Design review of the part built by this model. Coordinates are the model's own, in mm. A direction names the side the tool comes from. Give positions to 0.01 mm unless a question says otherwise; leave off trailing zeros. Order: outer loops, then holes, each group sorted by start corner. A loop starts at its lowest first (then second) coordinate and runs counter-clockwise, first axis right, second up.
```python
from build123d import *

# Parameters (mm, degrees)
F0_W     = 40
F0_H     = 36
F0_W_2   = 34
F0_H_2   = 30
F1_DEPTH = 36.35
F0_R     = 3
F2_DEPTH = 5
F3_R     = 5
F4_DEPTH = 40.001


with BuildPart() as f1:
    # F0 (on Top) → F1 (new body)
    with BuildSketch(Plane.XY):
        with Locations((3.016732, 5.513384)):
            Rectangle(F0_W, F0_H)
        with Locations((3.016732, 5.513384)):
            Rectangle(F0_W_2, F0_H_2, mode=Mode.SUBTRACT)
    extrude(amount=F1_DEPTH)

    # F0 (on Top) → F2 (join)
    with BuildSketch(Plane.XY):
        with Locations((3.016732, 5.513384)):
            Rectangle(F0_W, F0_H)
        with Locations((3.016732, 5.513384)):
            Rectangle(F0_W_2, F0_H_2, mode=Mode.SUBTRACT)
        with Locations((3.016732, 5.513384)):
            Rectangle(F0_W_2, F0_H_2)
        with Locations((3.016732, -4.486616)):
            Circle(F0_R, mode=Mode.SUBTRACT)
        with Locations((3.016732, 15.513384)):
            Circle(F0_R, mode=Mode.SUBTRACT)
    extrude(amount=F2_DEPTH)

    # F3 (on face) → F4 (cut, through all)
    with BuildSketch(Plane.YZ.offset(23.016732)):
        with Locations((5.513384, 10)):
            Circle(F3_R)
    extrude(amount=-F4_DEPTH, mode=Mode.SUBTRACT)


solid = f1.part
```
1. Take a section at C-C (y = -8.5). State the section outline as (x, z) points, then the cut area to 3 significant figures.
Recorded:
outline: (-16.98, 0) - (23.02, 0) - (23.02, 36.35) - (20.02, 36.35) - (20.02, 5) - (-13.98, 5) - (-13.98, 36.35) - (-16.98, 36.35) - close
area: 388 mm2
2. For line 1 along Y through (x, z) = (4.5, 28.5); line 2 along Y through (x, z) = (-15, 10); line 3 along X through (y, z) = (-1.5, 9), list the stretches that pass through material, from the lowest coordinate up.
Recorded:
line 1: y = -12.49 to -9.49, 20.51 to 23.51
line 2: y = -12.49 to 0.51, 10.51 to 23.51
line 3: x = -16.98 to -13.98, 20.02 to 23.02
3. For pin 1 (8 mm diameter, centred on x = 3.02, y = 15.51, fed in from +Z); pin 2 (10 mm diameter, centred on x = -2.5, y = 1, fed in from -Z), all flat-tipped, find the tip position at first contact; note any pin that passes through.
Recorded:
pin 1: stops at z = 5
pin 2: stops at z = 0
4. Take a section at A-A (z = 10). State the section outline as (x, y) points.
Recorded:
outline: (-16.98, -12.49) - (23.02, -12.49) - (23.02, 0.51) - (20.02, 0.51) - (20.02, -9.49) - (-13.98, -9.49) - (-13.98, 0.51) - (-16.98, 0.51) - close; (-16.98, 10.51) - (-13.98, 10.51) - (-13.98, 20.51) - (20.02, 20.51) - (20.02, 10.51) - (23.02, 10.51) - (23.02, 23.51) - (-16.98, 23.51) - close
5. Take a section at B-B (x = -11). State the section outline as (y, z) points, then the cut area to 3 significant figures.
Recorded:
outline: (-12.49, 0) - (23.51, 0) - (23.51, 36.35) - (20.51, 36.35) - (20.51, 5) - (-9.49, 5) - (-9.49, 36.35) - (-12.49, 36.35) - close
area: 368 mm2
6. Draft analysis for pull direction Y (two halves, no side actions). For faces 3 (the face through (-16.983, 5, 18)), 4 (the face through (2.366, 12.585, 2.465)), 5 (the face through (3, -12.487, 18)), state which applies: pulls with the +Y half, pulls with the -Y half, needs draft (parallel to the pull), parting line crosses it, or undercut.
Recorded:
face 3: needs draft
face 4: undercut
face 5: pulls with the -Y half
7. Take a section at D-D (z = 28.5). State the section outline as (x, y) points.
Recorded:
outline: (-16.98, -12.49) - (23.02, -12.49) - (23.02, 23.51) - (-16.98, 23.51) - close; hole (-13.98, -9.49) - (20.02, -9.49) - (20.02, 20.51) - (-13.98, 20.51) - close
8. Machinability: for faces 1 (the face through (3, -10, 36.35)), 2 (the face through (-13.983, 5, 20)), which of the approach directions +Z, -Z, +X, -X, +Y, -Y give a long, thin tool a straight path to every point of the face, cutting with its end or side? Answer none if there is none.
Recorded:
face 1: +Z, +X, -X, +Y, -Y
face 2: +Z
